Study the drawing (mm; zero at the part's minimum x, y, z) and answer. A direction names the side the tool comes from. Coordinates: 2 decimals unless noted, no trailing zeros. Loops run counter-clockwise (first coordinate to the right, second up) from the corner with the lowest first, then second, coordinate; pieces in that order, holes last. Notation, with made-up numbers: (-31, -36.75) - (-18, -36.75) arc R30 ccw to (-18, -0.75) - close; hole circle Ø7 at (55.5, 14). An arc over 180 degrees is marked (long way). One line per item, written item: value. Start each with the question number.
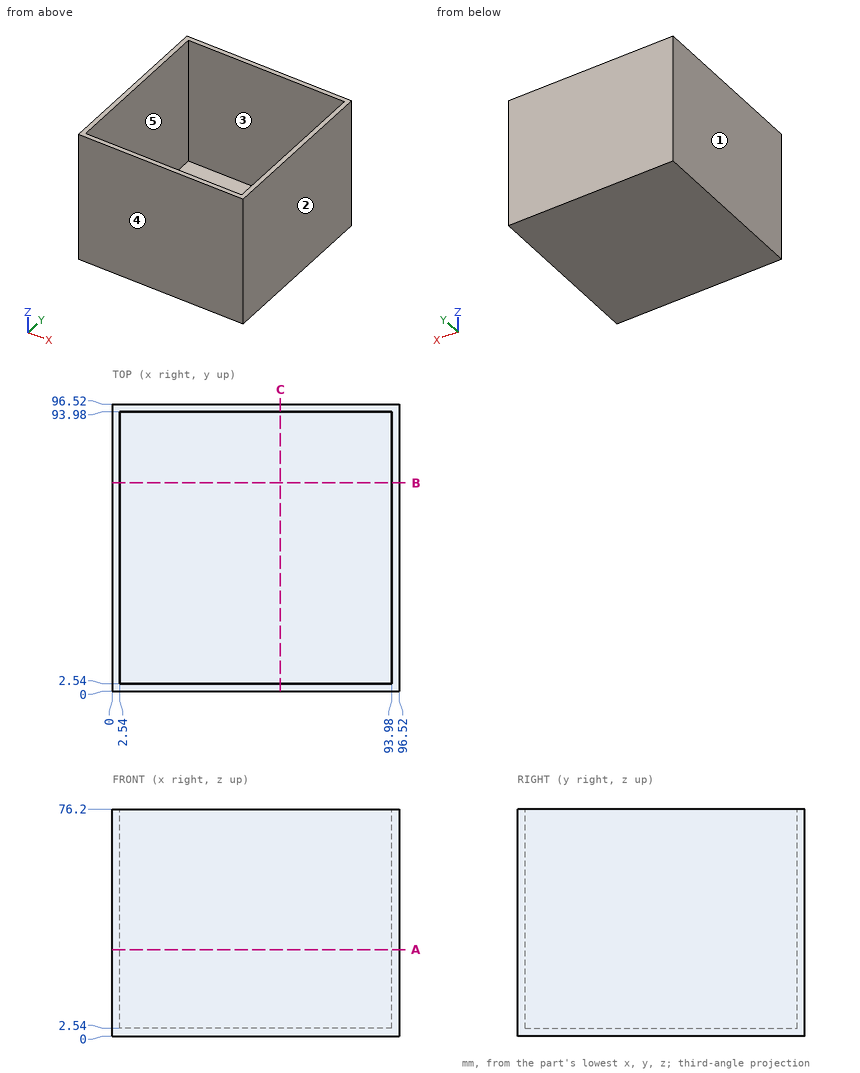
1) Section A-A, the plane z = 29 is taken. Determine the outline of the cut face in (x, y), and give its area (3 significant figures).
2) Straight lines are drawn through the part: L1, parallel to Y at x = 26, z = 52.5; L2, parallel to Z at x = 68.5, y = 62. For each, find the intervals that lie inside material, in ascending order.
3) Section B-B, the plane y = 70 is taken. Determine the outline of the cut face in (x, z), and give its area (3 significant figures).
4) Determine the mould class of the marked faces 1, 2 and 3 for opening direction X: released by +X, released by -X, zero draft, split by the parting line, or undercut.
5) For the marked faces 4 and 5, determine the directions among +Z, -Z, +X, -X, +Y, -Y from which every point of the face is accessible in a straight line to the end or side of a thin tool.
Answer below:
1. outline: (0, 0) - (96.52, 0) - (96.52, 96.52) - (0, 96.52) - close; hole (2.54, 2.54) - (93.98, 2.54) - (93.98, 93.98) - (2.54, 93.98) - close
1. area: 955 mm2
2. L1: 0 to 2.54, 93.98 to 96.52
2. L2: 0 to 2.54
3. outline: (0, 0) - (96.52, 0) - (96.52, 76.2) - (93.98, 76.2) - (93.98, 2.54) - (2.54, 2.54) - (2.54, 76.2) - (0, 76.2) - close
3. area: 619 mm2
4. face 1: released by -X
4. face 2: released by +X
4. face 3: undercut
5. face 4: +Z, -Z, +X, -X, -Y
5. face 5: +Z
